Here's how the part is built. I have some questions about the finished solid (model axes, mm). Face numbers are marked on the shaded views. A direction names the side the tool comes from. Round coordinates to 2 decimals unless told otherwise and drop trailing zeros. Loops run counter-clockwise (first coordinate to the right, second up) from the corner with the lowest first, then second, coordinate; pieces in that order, holes last. Notation, with made-up numbers: M 14,14.5 L 71,14.5 A10 ccw 71,33.5 Z; hole C -36,10 d2. An arc over 180 degrees is marked long. Answer as a JSON object with one key per item and string values.
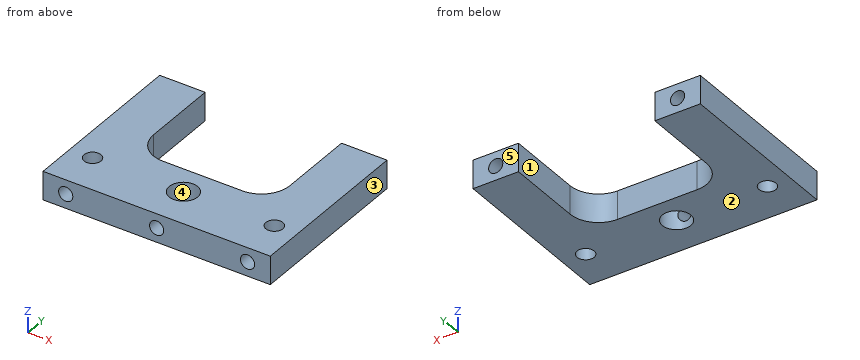
from build123d import *

# Parameters (mm, degrees)
F1_DEPTH       = 5
F2_R           = 5
F3_D           = 3
F6_D           = 2.5
F6_DEPTH       = 4.5
F6_TIP         = 0.7510757738
F6_ON_F5_D     = 2.5
F6_ON_F5_DEPTH = 4.5
F6_ON_F5_TIP   = 0.7510757738
F7_D           = 5
F8_D           = 2.5
F8_DEPTH       = 6
F8_TIP         = 0.7510757738


with BuildPart() as f1:
    # F0 (on Top) → F1 (new body)
    with BuildSketch(Plane.XY):
        Polygon((-20, -15.25), (20, -15.25), (20, 15.25), (12, 15.25), (12, -3.25), (-12, -3.25), (-12, 15.25), (-20, 15.25), align=None)
    extrude(amount=-F1_DEPTH)

    # F2
    f2_edges = [f1.edges().sort_by_distance(p)[0] for p in [
        (-12, -3.25, -2.5),
        (12, -3.25, -2.5),
    ]]
    fillet(f2_edges, radius=F2_R)

    # F3 (through all)
    with Locations(Plane.XY):
        with Locations((-16, -8.25), (16, -8.25)):
            Hole(F3_D / 2)

    # F6
    with Locations(Plane(origin=(0, 15.25, 0), x_dir=(-1, 0, 0), z_dir=(0, 1, 0))):
        with Locations((-16, -2.5), (16, -2.5)):
            Hole(F6_D / 2, depth=F6_DEPTH)
            with Locations((0, 0, -(F6_DEPTH + F6_TIP / 2))):  # 118° drill point
                Cone(0, F6_D / 2, F6_TIP, mode=Mode.SUBTRACT)

    # F6 on F5
    with Locations(Plane.XZ.offset(15.25)):
        with Locations((-16, -2.5), (16, -2.5)):
            Hole(F6_ON_F5_D / 2, depth=F6_ON_F5_DEPTH)
            with Locations((0, 0, -(F6_ON_F5_DEPTH + F6_ON_F5_TIP / 2))):  # 118° drill point
                Cone(0, F6_ON_F5_D / 2, F6_ON_F5_TIP, mode=Mode.SUBTRACT)

    # F7 (through all)
    with Locations(Plane.XY):
        with Locations((0, -8.25)):
            Hole(F7_D / 2)

    # F8
    with Locations(Plane.XZ.offset(15.25)):
        with Locations((0, -2.5)):
            Hole(F8_D / 2, depth=F8_DEPTH)
            with Locations((0, 0, -(F8_DEPTH + F8_TIP / 2))):  # 118° drill point
                Cone(0, F8_D / 2, F8_TIP, mode=Mode.SUBTRACT)


solid = f1.part
Item 1: I want a section at A-A on y = 7.5. List the corners of the cut face in (x, z) for me.
Solution:
{"outline": "M -20,-5 L -12,-5 L -12,0 L -20,0 Z; M 12,-5 L 20,-5 L 20,0 L 12,0 Z"}
Item 2: If I drill on L1, parallel to X at y = -13.7, z = -2.5; L2, parallel to X at y = 14.15, z = -2.5; L3, parallel to Z at x = -16, y = -13.9, over which ranges is the centre line in solid material (lowest first)? Write a range as from..to.
Solution:
{"L1": "x = -20..-17.25, -14.75..-1.25, 1.25..14.75, 17.25..20", "L2": "x = -20..-17.25, -14.75..-12, 12..14.75, 17.25..20", "L3": "z = -5..-3.75, -1.25..0"}
Item 3: We'd pull the mould along X, two halves only. Please class the marked faces 3, 4 and 5: +X half, -X half, draft (parallel to the pull), parting line (faces both ways), or undercut.
Solution:
{"face 3": "+X half", "face 4": "undercut", "face 5": "draft"}
Item 4: For the marked faces 1 and 2, which set-ups out of +Z, -Z, +X, -X, +Y, -Y let a thin tool reach every point of the face, with its end or its side?
Solution:
{"face 1": "+Z, -Z, +Y", "face 2": "-Z, +X, -X, +Y, -Y"}
Item 5: For P1, Ø5, axis at x = -10, y = 11.5, coming from the +Z side; P2, Ø1.5, axis at x = 16, z = -2.5, coming from the -Y side; P3, Ø2, axis at x = -16, z = -2.5, coming from the -Y side, each with a flat end and sliding along its axis, tell me the tip position at first contact or that it passes through.
Solution:
{"P1": "stops at z = 0", "P2": "stops at y = -10.45", "P3": "stops at y = -10.6"}
Item 6: I want a section at D-D on x = -5. List the corners of the cut face in (y, z) for me.
Solution:
{"outline": "M -15.25,-5 L -3.25,-5 L -3.25,0 L -15.25,0 Z"}
Item 7: I want a section at B-B on x = 0. List the corners of the cut face in (y, z) for me.
Solution:
{"outline": "M -15.25,-5 L -10.75,-5 L -10.75,-3.75 L -15.25,-3.75 Z; M -15.25,-1.25 L -10.75,-1.25 L -10.75,0 L -15.25,0 Z; M -5.75,-5 L -3.25,-5 L -3.25,0 L -5.75,0 Z"}
Item 8: I want a section at C-C on y = -8.25. List the corners of the cut face in (x, z) for me, plus the area to 3 significant figures.
Solution:
{"outline": "M -20,-5 L -17.5,-5 L -17.5,0 L -20,0 Z; M -14.5,-5 L -2.5,-5 L -2.5,0 L -14.5,0 Z; M 2.5,-5 L 14.5,-5 L 14.5,0 L 2.5,0 Z; M 17.5,-5 L 20,-5 L 20,0 L 17.5,0 Z", "area": "145 mm2"}
